For this review, use the dimensioned drawing (mm, ordinates from the lowest corner) and the shaded views. A direction names the side the tool comes from. Round coordinates to 2 decimals unless told otherwise and drop trailing zeros. Write each loop counter-clockwise with the first axis right and the second up, starting at its lowest first coordinate (ties: lowest second). Pieces come first, ordered by that corner, then holes. Notation, with made-up numbers: M -30.5,-19.5 L 18.5,-19.5 A23 cw 18.5,-0.5 Z; hole C 17,-34.75 d4. An arc over 180 degrees is marked long. Use one line per item in the form item = value. Start each with the question number.
Item 1: For P1, Ø10, axis at x = 6.5, z = 7.5, coming from the -Y side; P2, Ø0.8, axis at y = 1.5, z = 21, coming from the -X side (1 decimal), all flat-tipped, find the tip position at first contact; note any pin that passes through.
Item 2: Draft analysis for pull direction X (two halves, no side actions). For the marked faces 6, 7, 8 and 9, state which applies: released by +X, released by -X, zero draft, split by the parting line, or undercut.
Item 3: For the marked faces 1, 2, 3, 4 and 5, list the 3-axis set-ups (+Z, -Z, +X, -X, +Y, -Y) from which the entire face can be reached by the end or side of a thin tool; tool diameter is ignored.
Item 4: For line 1 (X direction, y = 2.1, z = 19.75); line 2 (X direction, y = 1.15, z = 13) (1 decimal); line 3 (X direction, y = 1.7, z = 19), list the stretches that pass through material, from the lowest coordinate up. Write a range as [from, to].
Item 5: Add section C-C (z = 19.25). State the section outline as (x, y) points.
Item 6: Add section D-D (x = 5). State the section outline as (y, z) points.
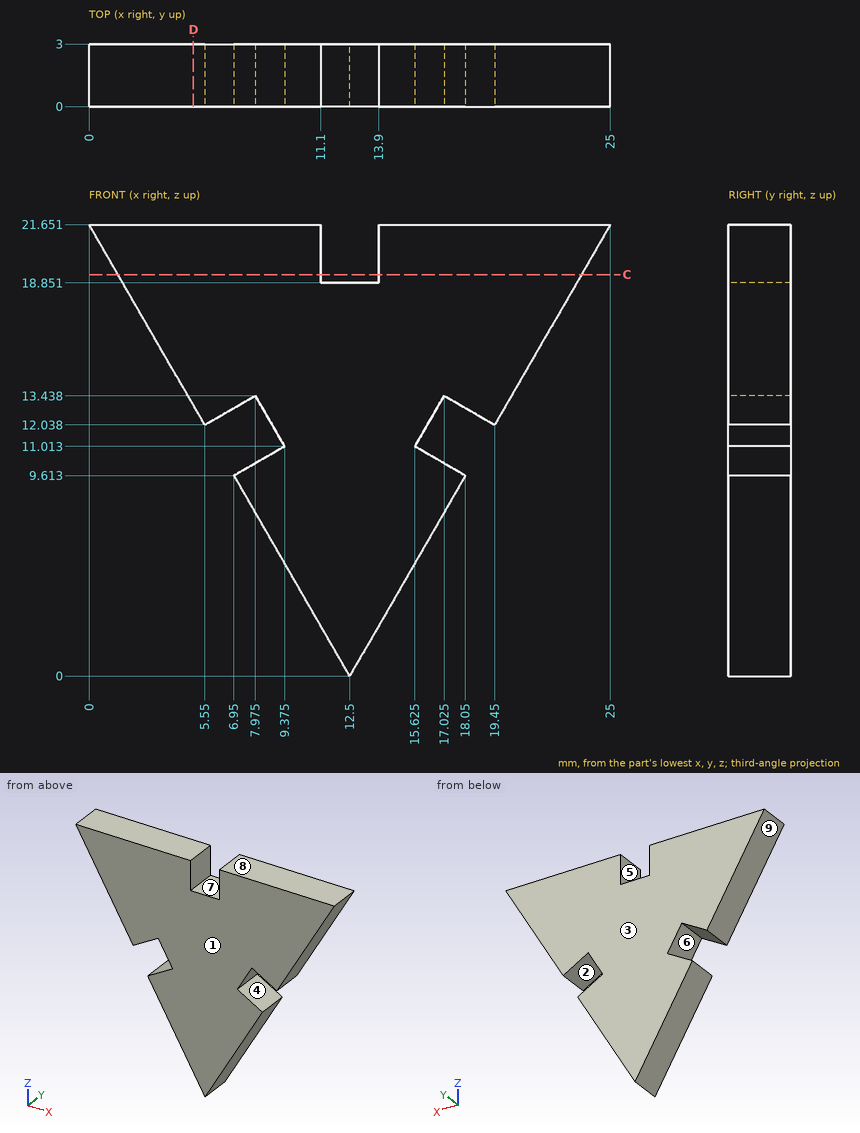
Calculated:
q1.P1 = 0
q1.P2 = 0.1
q2.face_6 = undercut
q2.face_7 = undercut
q2.face_8 = zero draft
q2.face_9 = released by -X
q3.face_1 = +Z, -Z, +X, -X, -Y
q3.face_2 = +Y, -Y
q3.face_3 = +Z, -Z, +X, -X, +Y
q3.face_4 = +X, +Y, -Y
q3.face_5 = +Z, +Y, -Y
q4.line_1 = [1.1, 11.1], [13.9, 23.9]
q4.line_2 = [5, 7.2], [8.2, 16.8], [17.8, 20]
q4.line_3 = [1.53, 11.1], [13.9, 23.47]
q5.outline = M 1.39,0 L 11.1,0 L 11.1,3 L 1.39,3 Z; M 13.9,0 L 23.61,0 L 23.61,3 L 13.9,3 Z
q6.outline = M 0,12.99 L 3,12.99 L 3,21.65 L 0,21.65 Z
